```python
from build123d import *

# Parameters (mm, degrees)
SKETCH1_W               = 139.7
SKETCH1_H               = 26.924
BOSS_EXTRUDE1_DEPTH     = 5.334
SKETCH2_W               = 38.1
SKETCH2_H               = 18.034
CUT_EXTRUDE1_DEPTH      = 104.832998003
SKETCH3_W               = 48.37176
SKETCH3_H               = 18.034
CUT_EXTRUDE3_DEPTH      = 104.832998003
SKETCH4_W               = 5.08
SKETCH4_H               = 5.08
CUT_EXTRUDE4_DEPTH      = 104.832998003
FILLET1_R               = 8.89
SKETCH5_W               = 8.89
SKETCH5_H               = 5.334
CUT_EXTRUDE5_DEPTH      = 104.832998003
SKETCH6_W               = 3.048
SKETCH6_H               = 8.89
CUT_EXTRUDE6_DEPTH      = 104.832998003
CUT_EXTRUDE7_DEPTH      = 104.832998003
CUT_EXTRUDE8_DEPTH      = 104.832998003
CUT_EXTRUDE9_DEPTH      = 104.832998003
CUT_EXTRUDE9_DEPTH_BACK = 104.832998003


with BuildPart() as part:
    # Sketch1 → Boss-Extrude1 (new body)
    with BuildSketch(Plane.XY):
        with Locations((32.120305114, 5.376704658)):
            Rectangle(SKETCH1_W, SKETCH1_H)
    extrude(amount=BOSS_EXTRUDE1_DEPTH)

    # Sketch2 → Cut-Extrude1 (cut, through all)
    with BuildSketch(Plane.XY.offset(5.334)):
        with Locations((-18.679694886, 9.821704658)):
            Rectangle(SKETCH2_W, SKETCH2_H)
    extrude(amount=-CUT_EXTRUDE1_DEPTH, mode=Mode.SUBTRACT)

    # Sketch3 → Cut-Extrude3 (cut, through all)
    with BuildSketch(Plane.XY.offset(5.334)):
        with Locations((49.956185114, 9.821704658)):
            Rectangle(SKETCH3_W, SKETCH3_H)
    extrude(amount=-CUT_EXTRUDE3_DEPTH, mode=Mode.SUBTRACT)

    # Sketch4 → Cut-Extrude4 (cut, through all)
    with BuildSketch(Plane.XY.offset(5.334)):
        with Locations((2.910305114, 16.298704658)):
            Rectangle(SKETCH4_W, SKETCH4_H)
    extrude(amount=-CUT_EXTRUDE4_DEPTH, mode=Mode.SUBTRACT)

    # Fillet1
    fillet1_edges = [part.edges().sort_by_distance(p)[0] for p in [
        (101.970305114, -8.085295342, 2.667),
    ]]
    fillet(fillet1_edges, radius=FILLET1_R)

    # Sketch5 → Cut-Extrude5 (cut, through all)
    with BuildSketch(Plane.XY.offset(5.334)):
        with Locations((14.975305114, 12.361704658)):
            Rectangle(SKETCH5_W, SKETCH5_H)
    extrude(amount=-CUT_EXTRUDE5_DEPTH, mode=Mode.SUBTRACT)

    # Sketch6 → Cut-Extrude6 (cut, through all)
    with BuildSketch(Plane.XY.offset(5.334)):
        with Locations((75.666065114, 5.249704658)):
            Rectangle(SKETCH6_W, SKETCH6_H)
    extrude(amount=-CUT_EXTRUDE6_DEPTH, mode=Mode.SUBTRACT)

    # Sketch7 → Cut-Extrude7 (cut, through all)
    with BuildSketch(Plane.XY.offset(5.334)):
        Polygon((77.190065114, 9.694704658), (74.142065114, 12.742704658), (74.142065114, 9.694704658), align=None)
    extrude(amount=-CUT_EXTRUDE7_DEPTH, mode=Mode.SUBTRACT)

    # Sketch8 → Cut-Extrude8 (cut, through all)
    with BuildSketch(Plane.XY.offset(5.334)):
        Polygon((0.370305114, 1.312704658), (3.418305114, 4.360704658), (3.418305114, 9.694704658), (0.370305114, 12.742704658), align=None)
    extrude(amount=-CUT_EXTRUDE8_DEPTH, mode=Mode.SUBTRACT)

    # Sketch9 → Cut-Extrude9 (cut, two sides: drawn at the far end of the back side and taken through both)
    with BuildSketch(Plane.XY.offset(5.334).offset(-CUT_EXTRUDE9_DEPTH_BACK)):
        Polygon((3.418305114, 0.804704658), (3.418305114, 4.360704658), (0.370305114, 1.312704658), (0.370305114, 0.804704658), align=None)
    extrude(amount=CUT_EXTRUDE9_DEPTH + CUT_EXTRUDE9_DEPTH_BACK, mode=Mode.SUBTRACT)


solid = part.part
```
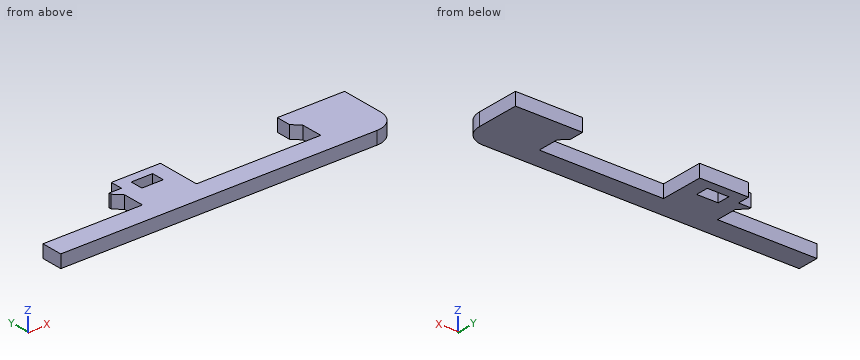
Here's how the part is built. I have some questions about the finished solid (model axes, mm). Coordinates: 2 decimals unless noted, no trailing zeros. Write each loop counter-clockwise with the first axis right and the second up, starting at its lowest first coordinate (ties: lowest second). Pieces come first, ordered by that corner, then holes. Notation, with made-up numbers: (82, 27.5) -> (122, 27.5) arc R34 cw to (122, 58.5) -> close; hole circle Ø4 at (19, 7.25). An arc over 180 degrees is marked (long way). Use a Markdown table: item, result. Add a question column.
(1) I'm going to push flat-ended pins straight in: P1, Ø1.1, axis at y = 13.5, z = 2, coming from the -X side; P2, Ø1.6, axis at x = -19.5, z = 1.5, coming from the +Y side; P3, Ø2.5, axis at y = 5, z = 3.5, coming from the -X side. Where does each tip first touch, or does it pass through?
(2) If we section it at C-C, the plane y = 4.25: Write out the boundary of the cut face in (x, z).
(3) If we section it at B-B, the plane z = 1.3: Write out the boundary of the cut face in (x, y).
(4) If we section it at A-A, the plane x = 15: Write out the boundary of the cut face in (y, z), and give its area (3 significant figures).
(5) Please list where these lines run through material, in increasing order: line 1 (X direction, y = 14, z = 2.7); line 2 (X direction, y = 5.25, z = 4.85); line 3 (X direction, y = 17.5, z = 0.9).
(6) If we section it at D-D, the plane y = 11.5: Write out the boundary of the cut face in (x, z), and give its area (3 significant figures).
Outcome:
| question | item | result |
|---|---|---|
| 1 | P1 | stops at x = 0.37 |
| 1 | P2 | stops at y = 0.8 |
| 1 | P3 | stops at x = 3.42 |
| 2 | outline | (3.42, 0) -> (25.77, 0) -> (25.77, 5.33) -> (3.42, 5.33) -> close; (77.19, 0) -> (101.97, 0) -> (101.97, 5.33) -> (77.19, 5.33) -> close |
| 3 | outline | (-37.73, -8.09) -> (93.08, -8.09) arc R8.89 ccw to (101.97, 0.8) -> (101.97, 18.84) -> (74.14, 18.84) -> (74.14, 12.74) -> (77.19, 9.69) -> (77.19, 0.8) -> (25.77, 0.8) -> (25.77, 18.84) -> (5.45, 18.84) -> (5.45, 13.76) -> (0.37, 13.76) -> (0.37, 12.74) -> (3.42, 9.69) -> (3.42, 0.8) -> (-37.73, 0.8) -> close; hole (10.53, 9.69) -> (19.42, 9.69) -> (19.42, 15.03) -> (10.53, 15.03) -> close |
| 4 | outline | (-8.09, 0) -> (9.69, 0) -> (9.69, 5.33) -> (-8.09, 5.33) -> close; (15.03, 0) -> (18.84, 0) -> (18.84, 5.33) -> (15.03, 5.33) -> close |
| 4 | area | 115 mm^2 |
| 5 | line 1 | x = 5.45 to 10.53, 19.42 to 25.77, 74.14 to 101.97 |
| 5 | line 2 | x = 3.42 to 25.77, 77.19 to 101.97 |
| 5 | line 3 | x = 5.45 to 25.77, 74.14 to 101.97 |
| 6 | outline | (1.61, 0) -> (10.53, 0) -> (10.53, 5.33) -> (1.61, 5.33) -> close; (19.42, 0) -> (25.77, 0) -> (25.77, 5.33) -> (19.42, 5.33) -> close; (75.38, 0) -> (101.97, 0) -> (101.97, 5.33) -> (75.38, 5.33) -> close |
| 6 | area | 223 mm^2 |
